Verification items for the finished model (mm, model axes). A direction names the side the tool comes from. Give positions to 0.01 mm unless a question says otherwise; leave off trailing zeros. Loops run counter-clockwise (first coordinate to the right, second up) from the corner with the lowest first, then second, coordinate; pieces in that order, holes last. Notation, with made-up numbers: (61.25, 36.5) - (118.25, 36.5) arc R29 ccw to (118.25, 59.5) - close; hole circle Ø5 at (57.25, 86.5). An arc over 180 degrees is marked (long way). One line per item, written item: value. Start each with the question number.
1. Sectioned sample at B-B (z = -7). Record the cut outline in (x, y), plus the area to 3 significant figures.
2. Access from +Z, -Z, +X, -X, +Y, -Y to the whole of each face (thin tool, end or side, straight path). Record for faces 1 (the flat face through (-21.817, 4.449, -6.224)), 2 (the cylindrical face through (-6.67, -21.17, -3.03)), 3 (the cylindrical face through (-7.25, -7.45, -6.35)).
3. Scan lines: L1, parallel to Z at x = -7.62, y = -15 (3 decimals); L2, parallel to X at y = -21.5, z = 0 (3 decimals); L3, parallel to Z at x = -27, y = 5.5. Record each from-to range of solid material in increasing order. Write a range as [from, to].
4. Sectioned sample at A-A (z = 0). Count the separate pieces of the cut face and the enclosed holes in it, plus the area to 3 significant figures.
5. Sectioned sample at C-C (y = -22). Record the cut outline in (x, z) (3 decimals), plus the area to 3 significant figures.
6. Mould release check, pull along Z, two halves, no side actions. Record for faces 4 (the cylindrical face through (13.61, 1.84, -2.75)), 5 (the cylindrical face through (-7.254, -7.438, 3.175)), 6 (the cylindrical face through (-7.99, -7.45, -6.35)): pulls with the +Z half, pulls with the -Z half, needs draft (parallel to the pull), parting line crosses it, or undercut.
7. Gauge pin test, flat ends, axial feed: pin 1 (10 mm diameter, centred on y = -2.5, z = 6, fed in from +X); pin 2 (10 mm diameter, centred on x = -6, z = 3.5, fed in from +Y); pin 3 (1.1 mm diameter, centred on x = -8, z = -2, fed in from -Y). Record the tip position at first contact, or that the pin passes through.
from build123d import *

# Parameters (mm, degrees)
SKETCH3_W          = 6.35
SKETCH3_H          = 25.4
SKETCH4_R          = 3.175
CUT_EXTRUDE1_DEPTH = 19.05
SKETCH6_R          = 3.175
CUT_EXTRUDE2_DEPTH = 25.4


with BuildPart() as part:
    # Sketch2 → Revolve1 (revolve)
    with BuildSketch(Plane.XY, mode=Mode.PRIVATE) as revolve1_sk:
        Polygon((5.230557596, 5.79531338), (1.09963978, 9.926231195), (5.589767841, 14.416359256), (3.254901249, 16.751225847), (-1.235226811, 12.261097787), (0.740429535, 10.28544144), (-12.729954646, -3.184942741), (-8.239826586, -7.675070802), align=None)
    revolve1 = revolve(revolve1_sk.sketch.rotate(Axis((-8.239826586, -7.675070802, 0), (0.7071067811865436, 0.7071067811865516, 0)), 180), axis=Axis((-8.239826586, -7.675070802, 0), (0.7071067811865436, 0.7071067811865516, 0)))

    # Mirror1: Revolve1 across plane
    add(revolve1.mirror(Plane(origin=(-7.62, 0, 0), x_dir=(0, 0, 1), z_dir=(1, 0, 0))))

    # Sketch3 → Revolve2 (revolve)
    with BuildSketch(Plane.XY, mode=Mode.PRIVATE) as revolve2_sk:
        with Locations((-4.445, -20.994897388)):
            Rectangle(SKETCH3_W, SKETCH3_H)
    revolve(revolve2_sk.sketch.rotate(Axis((-7.62, -8.294897388, 0), (0, -1, 0)), 90), axis=Axis((-7.62, -8.294897388, 0), (0, -1, 0)))

    # Sketch4 → Cut-Extrude1 (cut)
    with BuildSketch(Plane(origin=(-13.132935488, 13.132935488, 0), x_dir=(0, 0, 1), z_dir=(-0.7071067811865437, 0.7071067811865515, 0))):
        with Locations(Location((0, -10.376964701, 0), (0, 0, 270))):
            Circle(SKETCH4_R)
    cut_extrude1 = extrude(amount=-CUT_EXTRUDE1_DEPTH, mode=Mode.SUBTRACT)

    # Mirror2: Cut-Extrude1 across plane
    add(cut_extrude1.mirror(Plane(origin=(-7.62, 0, 0), x_dir=(0, 0, 1), z_dir=(1, 0, 0))), mode=Mode.SUBTRACT)

    # Sketch6 → Cut-Extrude2 (cut)
    with BuildSketch(Plane.XZ.offset(33.694897388)):
        with Locations(Location((-7.62, 0, 0), (0, 0, 270))):
            Circle(SKETCH6_R)
    extrude(amount=-CUT_EXTRUDE2_DEPTH, mode=Mode.SUBTRACT)


solid = part.part
Results are:
1. outline: (-29.12, 6.13) - (-24.63, 1.64) - (-16.31, 9.96) - (-20.8, 14.45) - close; (1.07, 9.96) - (9.39, 1.64) - (13.88, 6.13) - (5.56, 14.45) - close
1. area: 149 mm^2
2. face 1: none
2. face 2: -Y
2. face 3: -Z
3. L1: z = [-6.35, -3.175], [3.175, 6.35]
3. L2: x = [-13.97, -10.795], [-4.445, -1.27]
3. L3: z = [-7.77, -3.29], [3.29, 7.77]
4. separate pieces: 3
4. enclosed holes: 0
4. area: 429 mm^2
5. outline: circle Ø12.7 at (-7.62, 0); hole circle Ø6.35 at (-7.62, 0)
5. area: 95.0 mm^2
6. face 4: parting line crosses it
6. face 5: undercut
6. face 6: pulls with the -Z half
7. pin 1: stops at x = 13.21
7. pin 2: stops at y = 7.88
7. pin 3: stops at y = -4.14
